Can you work these out from the drawing? Everything is in mm from the part's minimum corner. Round coordinates to 2 decimals unless told otherwise and drop trailing zeros. Order: outer loops, then holes, each group sorted by start corner. A loop starts at its lowest first (then second) coordinate and runs counter-clockwise, first axis right, second up. Notation, with made-up numbers: M -26.5,64.25 L -22.5,64.25 A13 ccw -22.5,88.25 Z; hole C 21,19 d9. An arc over 180 degrees is marked long. Write each question's results on one line, items separated by ' | '. Start each with the question number.
1. Suppose I cut it at B-B on z = 4.25. Write out the boundary of the cut face in (x, y).
2. Suppose I cut it at A-A on y = 3. Write out the boundary of the cut face in (x, z) (1 decimal).
3. Please list where these lines run through material, in increasing order: L1, parallel to Z at x = 2.1, y = 2; L2, parallel to X at y = 3.75, z = 14.5; L3, parallel to X at y = 3.55, z = 5 (1 decimal).
4. We'd pull the mould along X, two halves only. Please class the marked faces 1, 2 and 3: released by +X, released by -X, zero draft, split by the parting line, or undercut.
5. I'm going to push flat-ended pins straight in: pin 1 (1.5 mm diameter, centred on x = 2, z = 4.5, fed in from +Y); pin 2 (1.1 mm diameter, centred on y = 2.5, z = 19.5, fed in from -X). Where does each tip first touch, or does it pass through?
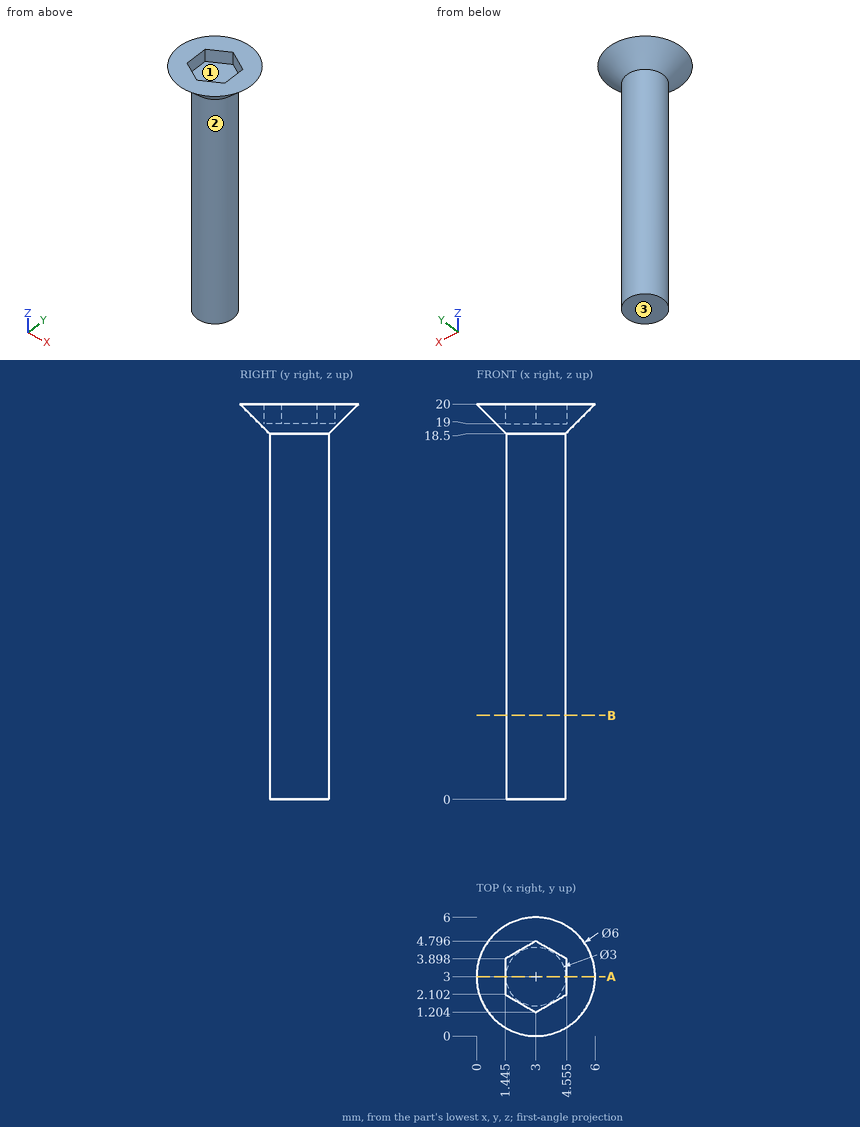
Filled sheet:
1) outline: C 3,3 d3
2) outline: M 0,20 L 1.5,18.5 L 1.5,0 L 4.5,0 L 4.5,18.5 L 6,20 L 4.6,20 L 4.6,19 L 1.4,19 L 1.4,20 Z
3) L1: z = 0 to 19 | L2: x = 1.7 to 4.3 | L3: x = 1.6 to 4.4
4) face 1: undercut | face 2: split by the parting line | face 3: zero draft
5) pin 1: stops at y = 4.48 | pin 2: stops at x = 0.01
